```python
from build123d import *

# Parameters (mm, degrees)
SCHIZZO1_R                   = 17.25
ESTRUSIONE_ESTRUSIONE1_DEPTH = 23.85
TAGLIO_ESTRUSIONE1_START     = -11.05
TAGLIO_ESTRUSIONE1_DEPTH     = 11.05
FORO_25_5_12_7_1_D           = 12.7
SCHIZZO5_R                   = 17.25
SCHIZZO5_R_2                 = 12.7
TAGLIO_ESTRUSIONE2_DEPTH     = 12.8


with BuildPart() as part:
    # Schizzo1 → Estrusione-Estrusione1 (new body)
    with BuildSketch(Plane.XY):
        Circle(SCHIZZO1_R)
    extrude(amount=ESTRUSIONE_ESTRUSIONE1_DEPTH)

    # Schizzo2 → Taglio-Estrusione1 (cut)
    with BuildSketch(Plane.XY.offset(23.85).offset(TAGLIO_ESTRUSIONE1_START)):
        with BuildLine():
            Line((-14.938938215, 8.625), (0, 17.25))
            ThreePointArc((0, 17.25), (-8.625, 14.938938215), (-14.938938215, 8.625))
        make_face()
        with BuildLine():
            Line((-14.938938215, -8.625), (-14.938938215, 8.625))
            ThreePointArc((-14.938938215, 8.625), (-17.25, 0), (-14.938938215, -8.625))
        make_face()
        with BuildLine():
            Line((0, -17.25), (-14.938938215, -8.625))
            ThreePointArc((-14.938938215, -8.625), (-8.625, -14.938938215), (0, -17.25))
        make_face()
        with BuildLine():
            ThreePointArc((0, -17.25), (8.625, -14.938938215), (14.938938215, -8.625))
            Line((14.938938215, -8.625), (0, -17.25))
        make_face()
        with BuildLine():
            ThreePointArc((17.25, 0), (16.662220503, 4.464628528), (14.938938215, 8.625))
            Line((14.938938215, 8.625), (14.938938215, -8.625))
            ThreePointArc((14.938938215, -8.625), (16.662220503, -4.464628528), (17.25, 0))
        make_face()
        with BuildLine():
            ThreePointArc((14.938938215, 8.625), (8.625, 14.938938215), (0, 17.25))
            Line((0, 17.25), (14.938938215, 8.625))
        make_face()
    extrude(amount=TAGLIO_ESTRUSIONE1_DEPTH, mode=Mode.SUBTRACT)

    # Foro Ø25.5 (12.7)-1 (through all)
    with Locations(Plane.XY.offset(23.85)):
        with Locations((0, 0)):
            Hole(FORO_25_5_12_7_1_D / 2)

    # Schizzo5 → Taglio-Estrusione2 (cut)
    with BuildSketch(Plane(origin=(0, 0, 0), x_dir=(-1, 0, 0), z_dir=(0, 0, -1))):
        Circle(SCHIZZO5_R)
        Circle(SCHIZZO5_R_2, mode=Mode.SUBTRACT)
    extrude(amount=-TAGLIO_ESTRUSIONE2_DEPTH, mode=Mode.SUBTRACT)


solid = part.part
```
Can you work these out from the model? Positions are in its coordinate system, mm. A direction names the side the tool comes from. Round coordinates to 2 decimals unless told otherwise and drop trailing zeros. Loops run counter-clockwise (first coordinate to the right, second up) from the corner with the lowest first, then second, coordinate; pieces in that order, holes last. Notation, with made-up numbers: M 7.25,89.25 L 18.25,89.25 A24 cw 18.25,114.25 Z; hole C -15,1 d8. An arc over 180 degrees is marked long. Answer as a JSON object with one key per item and string values. Group by question number.
Q1. Imagine slicing it at A-A, the plane y = 0. Please give me the cut outline in (x, z).
Q2. Please list where these lines run through material, in increasing order: L1, parallel to Y at x = 0, z = 14; L2, parallel to Y at x = 1, z = 14.5; L3, parallel to X at y = -2, z = 16.
Q3. Imagine slicing it at C-C, the plane x = 10.5. Please give me the cut outline in (y, z).
Q4. We'd pull the mould along X, two halves only. Please class faces 3 (the cylindrical face through (2.75, -12.4, 6.31)), 4 (the cylindrical face through (1.38, -6.2, 11.76)), 5 (the flat face through (-7.57, 12.88, 18.25)): +X half, -X half, draft (parallel to the pull), parting line (faces both ways), or undercut.
Q5. On a 3-axis mill with a long thin cutter (end or side, diameter ignored), from which of +Z, -Z, +X, -X, +Y, -Y can I reach the whole of each face in a straight line? I mean faces 1 (the flat face through (0, -7, 23.85)), 2 (the flat face through (1, -13, 12.8)). Say none if no direction works.
Q6. Imagine slicing it at D-D, the plane y = -4.5. Please give me the cut outline in (x, z), then the cut area to 3 significant figures.
Q7. Imagine slicing it at B-B, the plane z = 19.5. Please give me the cut outline in (x, y) (3 decimals).
Q8. Will these pins go through, and if not, where does the flat tip stop? pin 1 (8 mm diameter, centred on x = 5.5, z = 4.5, fed in from +Y); pin 2 (8 mm diameter, centred on x = 0.5, z = 4.5, fed in from +Y); pin 3 (12 mm diameter, centred on x = -1.5, y = 12.5, fed in from -Z); pin 4 (10 mm diameter, centred on x = 0, y = 0, fed in from -Z).
Findings:
{
 "1": {"outline": "M -14.94,12.8 L -12.7,12.8 L -12.7,0 L -6.35,0 L -6.35,23.85 L -14.94,23.85 Z; M 6.35,0 L 12.7,0 L 12.7,12.8 L 14.94,12.8 L 14.94,23.85 L 6.35,23.85 Z"},
 "2": {"L1": "y = -17.25 to -6.35, 6.35 to 17.25", "L2": "y = -16.67 to -6.27, 6.27 to 16.67", "L3": "x = -14.94 to -6.03, 6.03 to 14.94"},
 "3": {"outline": "M -11.19,12.8 L -7.14,12.8 L -7.14,0 L 7.14,0 L 7.14,12.8 L 11.19,12.8 L 11.19,23.85 L -11.19,23.85 Z"},
 "4": {"face 3": "parting line", "face 4": "undercut", "face 5": "-X half"},
 "5": {"face 1": "+Z, +X, -X, +Y, -Y", "face 2": "-Z"},
 "6": {"outline": "M -14.94,12.8 L -11.88,12.8 L -11.88,0 L -4.48,0 L -4.48,23.85 L -14.94,23.85 Z; M 4.48,0 L 11.88,0 L 11.88,12.8 L 14.94,12.8 L 14.94,23.85 L 4.48,23.85 Z", "area": "420 mm2"},
 "7": {"outline": "M -14.939,-8.625 L 0,-17.25 L 14.939,-8.625 L 14.939,8.625 L 0,17.25 L -14.939,8.625 Z; hole C 0,0 d12.7"},
 "8": {"pin 1": "stops at y = 12.61", "pin 2": "stops at y = 12.7", "pin 3": "stops at z = 0", "pin 4": "passes through"}
}
